```python
from build123d import *

# Parameters (mm, degrees)
SKETCH_1_R      = 30
EXTRUDE_1_DEPTH = 90
SKETCH_2_R      = 40
EXTRUDE_2_DEPTH = 10
EXTRUDE_START   = 10
SKETCH_3_R      = 40
EXTRUDE_3_DEPTH = 10
SCALE_1_SCALE   = 0.345


with BuildPart() as part:
    # 草图1 → 凸台-拉伸1 (new body)
    with BuildSketch(Plane.XY):
        with Locations(Location((0, 0, 0), (0, 0, 180))):
            Circle(SKETCH_1_R)
    extrude(amount=EXTRUDE_1_DEPTH)

    # 草图2 → 凸台-拉伸2 (add)
    with BuildSketch(Plane.XY.offset(90)):
        Circle(SKETCH_2_R)
    extrude(amount=EXTRUDE_2_DEPTH)

    # 草图3 → 凸台-拉伸3 (add)
    with BuildSketch(Plane(origin=(0, 0, 0), x_dir=(-1, 0, 0), z_dir=(0, 0, -1)).offset(EXTRUDE_START)):
        with Locations(Location((0, 0, 0), (0, 0, 180))):
            Circle(SKETCH_3_R)
    extrude(amount=-EXTRUDE_3_DEPTH)


with BuildPart() as part_1:
    # 缩放比例1: scaled about (0, 0, 0)
    add(part.part.scale(SCALE_1_SCALE))


solid = part_1.part
```
Work out the finished part from the listing and answer in its coordinate system (mm). A direction names the side the tool comes from. Coordinates: 2 decimals unless noted, no trailing zeros. Loops run counter-clockwise (first coordinate to the right, second up) from the corner with the lowest first, then second, coordinate; pieces in that order, holes last.
1) Flat-ended cylindrical pins translate along their axes: pin 1 (10 mm diameter, centred on x = 4.5, z = 3, fed in from -Y); pin 2 (4 mm diameter, centred on x = 2.5, z = 15.5, fed in from +Y); pin 3 (1 mm diameter, centred on x = 4.5, z = 7.5, fed in from +Y). Find the tip coordinate at first contact, or state that the pin passes through.
Results:
pin 1: stops at y = -13.79
pin 2: stops at y = 10.34
pin 3: stops at y = 9.55
2) Consider probe 1 along Z at (x, y) = (-7, -11.75); probe 2 along X at (y, z) = (5.5, 31); probe 3 along Y at (x, z) = (-9.25, 20.5). Determine where each line is inside the solid, lowest interval first.
Results:
probe 1: z = -3.45 to 0, 31.05 to 34.5
probe 2: x = -8.77 to 8.77
probe 3: y = -4.64 to 4.64
3) Section D-D (z = 14.5) is taken. Give the vertices of the cut face in (x, y).
Results:
outline: circle Ø20.7 at (0, 0)
4) Section B-B (y = 11.5) is taken. Give the vertices of the cut face in (x, z).
Results:
outline: (-7.63, -3.45) - (7.63, -3.45) - (7.63, 0) - (-7.63, 0) - close; (-7.63, 31.05) - (7.63, 31.05) - (7.63, 34.5) - (-7.63, 34.5) - close
5) Section A-A (y = 0) is taken. Give the vertices of the cut face in (x, z).
Results:
outline: (-13.8, -3.45) - (13.8, -3.45) - (13.8, 0) - (10.35, 0) - (10.35, 31.05) - (13.8, 31.05) - (13.8, 34.5) - (-13.8, 34.5) - (-13.8, 31.05) - (-10.35, 31.05) - (-10.35, 0) - (-13.8, 0) - close
6) For faces 5 (the flat face through (5, -9.3, 0)), 6 (the cylindrical face through (-10.17, -9.33, -1.75)), determine the directions among +Z, -Z, +X, -X, +Y, -Y from which every point of the face is accessible in a straight line to the end or side of a thin tool.
Results:
face 5: none
face 6: +Z, -Z
7) For a pull along Z with two mould halves and no side action, classify faces 1 (the flat face through (0, 0, -3.45)), 2 (the flat face through (5, 9.3, 31.05)), 3 (the flat face through (0, 0, 34.5)), 4 (the cylindrical face through (-9.87, -3.11, 15.31)) as +Z half, -Z half, draft (parallel to the pull), parting line (faces both ways), or undercut.
Results:
face 1: -Z half
face 2: undercut
face 3: +Z half
face 4: undercut
